from build123d import *

# Parameters (mm, degrees)
F1_DEPTH = 20
F3_T     = -2


with BuildPart() as f1:
    # F0 (on Front) → F1 (new body)
    with BuildSketch(Plane.XZ):
        Polygon((0, 86.7171336596), (0, 0), (40, 0), (26.6733877361, 21.1794357747), (31.5282256901, 21.1794357747), (18.2016134262, 42.3588715494), (23.0564513803, 42.3588715494), (9.7298391163, 63.5383073241), (14.5846770704, 63.5383073241), align=None)
    extrude(amount=F1_DEPTH)

    # F2: F1 across plane


with BuildPart() as f1_1:
    add(f1.part)
    add(f1.part.mirror(Plane.YZ))

    # F3
    f3_openings = [f1_1.faces().sort_by_distance(p)[0] for p in [
        (0, -10, 0),
    ]]
    offset(amount=F3_T, openings=f3_openings, kind=Kind.INTERSECTION)


solid = f1_1.part
Geometry check sheet. Reference: the model listing, model coordinates, mm. A direction names the side the tool comes from. Coordinates: 2 decimals unless noted, no trailing zeros. Order: outer loops, then holes, each group sorted by start corner. A loop starts at its lowest first (then second) coordinate and runs counter-clockwise, first axis right, second up. Notation, with made-up numbers: (65, -29) - (98, -29) arc R30 ccw to (98, -2) - close; hole circle Ø2 at (55.5, 87.25). An arc over 180 degrees is marked (long way). Answer in a Markdown table with one row per item. Add a question column.
1) Cross-section at D-D, the plane x = -1.5. Record the cut outline in (y, z).
2) Gauge pin test, flat ends, axial feed: P1, Ø5.5, axis at x = 8, y = -14, coming from the +Z side; P2, Ø4, axis at x = -11.5, y = -5, coming from the -Z side; P3, Ø1.5, axis at x = -21, y = -7.5, coming from the -Z side. Record the tip position at first contact, or that the pin passes through.
3) Release check for a two-part mould opening along Z. For faces 1 (the flat face through (-30.447, -9.888, 11.427)), 2 (the flat face through (-33.43, -9.86, 10.44)), 3 (the flat face through (-7.39, -9.86, 74.97)) record: +Z half, -Z half, draft (parallel to the pull), parting line (faces both ways), or undercut.
4) Cross-section at A-A, the plane x = -21. Record the cut outline in (y, z), then the cut area to 3 significant figures.
5) Set-up check for faces 4 (the flat face through (-12, -10, 63.538)), 5 (the flat face through (-9, -10, 65.538)), 6 (the flat face through (21, -10, 42.359)): record each of +Z, -Z, +X, -X, +Y, -Y from which the full face is reachable in a straight line by a thin tool's end or side.
6) Material ranges on line 1 along Y through (x, z) = (20, 35.5); line 2 along X through (y, z) = (-13.25, 66.5); line 3 along X through (y, z) = (-16.25, 5), recorded low to high. Write a range as [from, to].
7) Cross-section at B-B, the plane z = 60. Record the cut outline in (x, y), then the cut area to 3 significant figures.
Check result:
| question | item | result |
|---|---|---|
| 1 | outline | (-20, 0) - (-18, 0) - (-18, 80.58) - (-2, 80.58) - (-2, 0) - (0, 0) - (0, 84.33) - (-20, 84.33) - close |
| 2 | P1 | stops at z = 78.37 |
| 2 | P2 | stops at z = 53.79 |
| 2 | P3 | stops at z = 32.96 |
| 3 | face 1 | -Z half |
| 3 | face 2 | undercut |
| 3 | face 3 | +Z half |
| 4 | outline | (-20, 0) - (-18, 0) - (-18, 34.16) - (-2, 34.16) - (-2, 0) - (0, 0) - (0, 37.91) - (-20, 37.91) - close; (-20, 42.36) - (0, 42.36) - (0, 45.63) - (-20, 45.63) - close |
| 4 | area | 277 mm² |
| 5 | face 4 | -X, +Y, -Y |
| 5 | face 5 | none |
| 5 | face 6 | +X, +Y, -Y |
| 6 | line 1 | y = [-20, -18], [-2, 0] |
| 6 | line 2 | x = [-12.72, -10.36], [10.36, 12.72] |
| 6 | line 3 | x = [-36.85, -34.49], [34.49, 36.85] |
| 7 | outline | (-11.96, -20) - (11.96, -20) - (11.96, 0) - (-11.96, 0) - close; hole (-9.59, -18) - (9.59, -18) - (9.59, -2) - (-9.59, -2) - close |
| 7 | area | 171 mm² |
